Can you work these out from the model? Positions are in its coordinate system, mm. Face numbers are marked on the shaded views. Round coordinates to 2 decimals unless told otherwise and drop trailing zeros. Order: outer loops, then holes, each group sorted by start corner. A loop starts at its lowest first (then second) coordinate and runs counter-clockwise, first axis right, second up. Notation, with made-up numbers: M -24.75,49.25 L 10.25,49.25 A21 cw 10.25,73.25 Z; hole C 48.25,53 d4. An arc over 180 degrees is marked long. One line per question, with ' | ' between items.
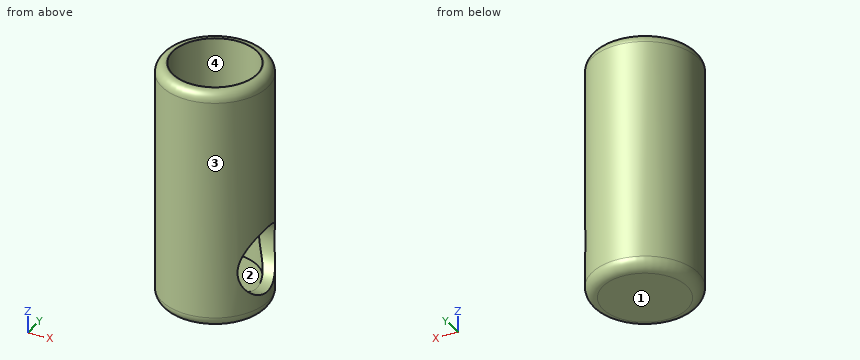
```python
from build123d import *

# Parameters (mm, degrees)
SKETCH002_R  = 3
PAD002_DEPTH = 10
SKETCH_R     = 4.825
SKETCH_R_2   = 3.825
PAD_DEPTH    = 20
SKETCH001_R  = 4.825
PAD001_DEPTH = 2
FILLET_R     = 1
FILLET001_R  = 0.9


with BuildPart() as body001:
    # Sketch002 → Pad002 (new body)
    with BuildSketch(Plane.YZ):
        with Locations((0, 3)):
            Circle(SKETCH002_R)
    extrude(amount=PAD002_DEPTH)


with BuildPart() as body:
    # Sketch → Pad (new body)
    with BuildSketch(Plane.XY):
        Circle(SKETCH_R)
        Circle(SKETCH_R_2, mode=Mode.SUBTRACT)
    extrude(amount=PAD_DEPTH)

    # Sketch001 (on Face3 of Pad) → Pad001 (join)
    with BuildSketch(Plane(origin=(0, 0, 0), x_dir=(1, 0, 0), z_dir=(0, 0, -1))):
        Circle(SKETCH001_R)
    extrude(amount=PAD001_DEPTH)

    # Boolean: cut Body001
    add(body001.part, mode=Mode.SUBTRACT)

    # Fillet
    fillet_edges = [body.edges().sort_by_distance(p)[0] for p in [
        (-4.825, 0, -2),
    ]]
    fillet(fillet_edges, radius=FILLET_R)

    # Fillet001
    fillet001_edges = [body.edges().sort_by_distance(p)[0] for p in [
        (-4.825, 0, 20),
    ]]
    fillet(fillet001_edges, radius=FILLET001_R)


solid = body.part
```
(1) If we section it at C-C on z = 3: Please give me the cut outline in (x, y) (3 decimals).
Final values:
outline: M 2.373,-3 A3.825 cw long 2.373,3 L 3.779,3 A4.825 ccw long 3.779,-3 Z
(2) If we section it at A-A on x = 0: Please give me the cut outline in (y, z) (3 decimals).
Final values:
outline: M -4.825,-1 A1 ccw -3.825,-2 L 3.825,-2 A1 ccw 4.825,-1 L 4.825,19.1 A0.9 ccw 3.925,20 L 3.825,20 L 3.825,0 L -3.825,0 L -3.825,20 L -3.925,20 A0.9 ccw -4.825,19.1 Z
(3) If we section it at B-B on z = 9: Please give me the cut outline in (x, y) (3 decimals), plus the area to 3 significant figures.
Final values:
outline: C 0,0 d9.65; hole C 0,0 d7.65 | area: 27.2 mm^2
(4) Will these pins go through, and if not, where does the flat tip stop? pin 1 Ø1.5 at (x, z) = (-2, 10.5) entering from +Y; pin 2 Ø4 at (x, y) = (-3.5, 0) entering from +Z; pin 3 Ø1.5 at (x, z) = (-1, 9) entering from +Y.
Final values:
pin 1: y = 4.66 | pin 2: z = 20 | pin 3: y = 4.82
(5) Thinking about a two-plate mould opening in X: for the marked faces 1, 2, 3 and 4, which applies, released by +X, released by -X, zero draft, split by the parting line, or undercut?
Final values:
face 1: zero draft | face 2: undercut | face 3: split by the parting line | face 4: undercut
(6) Please list where these lines run through material, in increasing order: probe 1 along Z at (x, y) = (0, 2.5); probe 2 along X at (y, z) = (-3.5, 9.5); probe 3 along Y at (x, z) = (3.15, 3). Write a range as [from, to].
Final values:
probe 1: [-2, 0] | probe 2: [-3.32, -1.54], [1.54, 3.32] | probe 3: [-3.65, -3], [3, 3.65]
